from build123d import *

# Parameters (mm, degrees)
F0_R     = 1.6
F1_DEPTH = 3
F2_T     = -1.5
F3_W     = 30
F3_H     = 44
F4_DEPTH = 1.501
F5_SIZE  = 1.55


with BuildPart() as f1:
    # F0 (on Top) → F1 (new body)
    with BuildSketch(Plane.XY):
        with BuildLine():
            Line((-12.9, -55.5), (17.9, -55.5))
            ThreePointArc((17.9, -55.5), (20.02132, -54.62132), (20.9, -52.5))
            Line((20.9, -52.5), (20.9, 47.5))
            ThreePointArc((20.9, 47.5), (18.556854, 53.156854), (12.9, 55.5))
            Line((12.9, 55.5), (-17.9, 55.5))
            ThreePointArc((-17.9, 55.5), (-20.02132, 54.62132), (-20.9, 52.5))
            Line((-20.9, 52.5), (-20.9, -47.5))
            ThreePointArc((-20.9, -47.5), (-18.556854, -53.156854), (-12.9, -55.5))
        make_face()
        with Locations((-16.081981, -50.681981)):
            Circle(F0_R, mode=Mode.SUBTRACT)
        with Locations((16.081981, 50.681981)):
            Circle(F0_R, mode=Mode.SUBTRACT)
    extrude(amount=F1_DEPTH)

    # F2
    f2_openings = [f1.faces().sort_by_distance(p)[0] for p in [
        (0, 0, 3),
    ]]
    offset(amount=F2_T, openings=f2_openings)

    # F3 (on face) → F4 (cut, through all)
    with BuildSketch(Plane.XY.offset(1.5)):
        Rectangle(F3_W, F3_H)
    extrude(amount=-F4_DEPTH, mode=Mode.SUBTRACT)

    # F5
    f5_edges = [f1.edges().sort_by_distance(p)[0] for p in [
        (14.481981, 50.681981, 0),
        (-17.681981, -50.681981, 0),
    ]]
    chamfer(f5_edges, length=F5_SIZE)


solid = f1.part
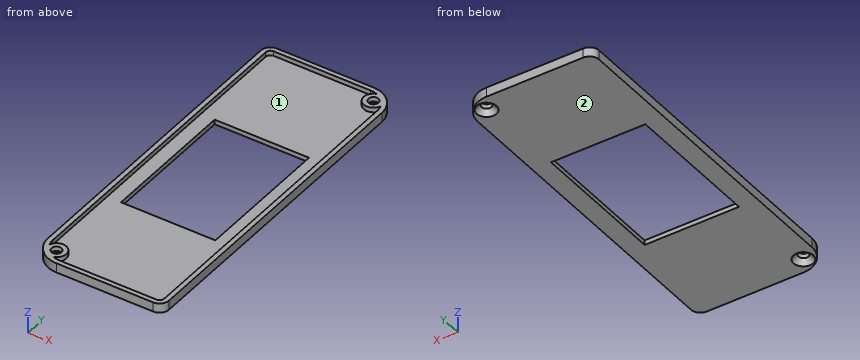
Input: part model. Units: mm. Frame: model coordinates. Face numbers are marked on the shaded views. Give positions to 0.01 mm unless a question says otherwise; leave off trailing zeros. Write each loop counter-clockwise with the first axis right and the second up, starting at its lowest first coordinate (ties: lowest second). Pieces come first, ordered by that corner, then holes. Notation, with made-up numbers: M 39.25,4.25 L 70.25,4.25 A14 cw 70.25,30.25 Z; hole C 61.5,89 d6. An arc over 180 degrees is marked long. Use one line per item in the form item = value.
1. Cut plane B-B on x = 8. Return loops of the section in (y, z).
Outcome:
outline = M -55.5,0 L -22,0 L -22,1.5 L -54,1.5 L -54,3 L -55.5,3 Z; M 22,0 L 55.5,0 L 55.5,3 L 54,3 L 54,1.5 L 22,1.5 Z
2. First-contact query: P1, Ø3, axis at x = -3, y = -34.5, coming from the +Z side; P2, Ø4, axis at x = -16.08, y = -50.68, coming from the -Z side. Flat tips, straight axial feed; report the tip coordinate or a pass-through.
Outcome:
P1 = 1.5
P2 = 1.15
3. Mould query, pull axis Y, two halves, no side actions, for the marked faces 1 and 2. Classes: released by +Y, released by -Y, zero draft, split by the parting line, or undercut.
Outcome:
face_1 = undercut
face_2 = zero draft
4. Cut plane D-D on y = -26.5. Return loops of the section in (x, z).
Outcome:
outline = M -20.9,0 L 20.9,0 L 20.9,3 L 19.4,3 L 19.4,1.5 L -19.4,1.5 L -19.4,3 L -20.9,3 Z
5. Ray query, L1, parallel to Y at x = 8, z = 1.7; L2, parallel to X at y = -6, z = 2.3; L3, parallel to X at y = -4, z = 0.9. Return the intervals inside material, ascending.
Outcome:
L1 = -55.5 to -54, 54 to 55.5
L2 = -20.9 to -19.4, 19.4 to 20.9
L3 = -20.9 to -15, 15 to 20.9
6. Cut plane A-A on y = 9. Return loops of the section in (x, z).
Outcome:
outline = M -20.9,0 L -15,0 L -15,1.5 L -19.4,1.5 L -19.4,3 L -20.9,3 Z; M 15,0 L 20.9,0 L 20.9,3 L 19.4,3 L 19.4,1.5 L 15,1.5 Z
7. Cut plane C-C on z = 0.9. Return loops of the section in (x, y), and give its area (3 significant figures).
Outcome:
outline = M -20.9,-47.5 A8 ccw -12.9,-55.5 L 17.9,-55.5 A3 ccw 20.9,-52.5 L 20.9,47.5 A8 ccw 12.9,55.5 L -17.9,55.5 A3 ccw -20.9,52.5 Z; hole C -16.08,-50.68 d4.5; hole M -15,-22 L 15,-22 L 15,22 L -15,22 Z; hole C 16.08,50.68 d4.5
area = 3,260 mm²
